from build123d import *

# Parameters (mm, degrees)
SKETCH1_R           = 11
BOSS_EXTRUDE1_DEPTH = 7
SKETCH2_R           = 11
BOSS_EXTRUDE2_DEPTH = 1
SKETCH3_R           = 13.5
SKETCH3_R_2         = 11
BOSS_EXTRUDE3_DEPTH = 1


with BuildPart() as part:
    # Sketch1 → Boss-Extrude1 (new body)
    with BuildSketch(Plane.XY):
        with BuildLine():
            ThreePointArc((0, -13.5), (13.5, 0), (0, 13.5))
            Line((0, 13.5), (-0.244738618, 13.497781411))
            Line((-0.244738618, 13.497781411), (-25, 13.273371546))
            ThreePointArc((-25, 13.273371546), (-38.377486998, -0.287261592), (-24.877625663, -13.726073795))
            Line((-24.877625663, -13.726073795), (-24.632285191, -13.723844279))
            Line((-24.632285191, -13.723844279), (0, -13.5))
        make_face()
        with Locations((-24.877625663, -0.226073795)):
            Circle(SKETCH1_R, mode=Mode.SUBTRACT)
        Circle(SKETCH1_R, mode=Mode.SUBTRACT)
    extrude(amount=BOSS_EXTRUDE1_DEPTH)

    # Sketch2 → Boss-Extrude2 (add)
    with BuildSketch(Plane(origin=(0, 0, 0), x_dir=(-1, 0, 0), z_dir=(0, 0, -1))):
        with Locations((24.877625663, -0.226073795)):
            Circle(SKETCH2_R)
    extrude(amount=-BOSS_EXTRUDE2_DEPTH)

    # Sketch3 → Boss-Extrude3 (add)
    with BuildSketch(Plane.XY.offset(7)):
        with Locations(Location((-24.877625663, -0.226073795, 0), (0, 0, 90.519379929))):
            Circle(SKETCH3_R)
        with Locations(Location((-24.877625663, -0.226073795, 0), (0, 0, 180))):
            Circle(SKETCH3_R_2, mode=Mode.SUBTRACT)
    extrude(amount=BOSS_EXTRUDE3_DEPTH)


solid = part.part
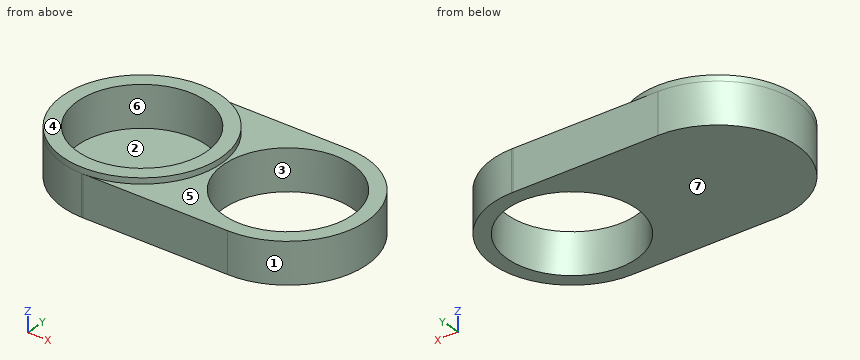
Verification items for the finished model (mm, model axes). Face numbers are marked on the shaded views. A direction names the side the tool comes from. Round coordinates to 2 decimals unless told otherwise and drop trailing zeros. Loops run counter-clockwise (first coordinate to the right, second up) from the corner with the lowest first, then second, coordinate; pieces in that order, holes last. Notation, with made-up numbers: (23.5, 39.25) - (70.5, 39.25) arc R20 cw to (70.5, 46.25) - close; hole circle Ø4 at (31, 71.5). An arc over 180 degrees is marked (long way). Use a Markdown table: item, result. Add a question column.
1. Section check D-D, the plane x = 10. Record the boundary of the cut face in (y, z).
2. Section check A-A, the plane x = -9. Record the boundary of the cut face in (y, z), plus the area to 3 significant figures.
3. Thickness scan on probe 1 along X at (y, z) = (-8.75, 1.25); probe 2 along X at (y, z) = (-1.25, 6.75); probe 3 along X at (y, z) = (0.25, 0.5). Record the ranges inside material, lowest first. Write a range as [from, to].
4. Section check C-C, the plane z = 2. Record the boundary of the cut face in (x, y).
5. Release check for a two-part mould opening along X. For the marked faces 1, 2, 3 and 4 record: released by +X, released by -X, zero draft, split by the parting line, or undercut.
6. Gauge pin test, flat ends, axial feed: pin 1 (1 mm diameter, centred on x = -11.5, z = 2.5, fed in from -Y); pin 2 (1.5 mm diameter, centred on y = -9, z = 4, fed in from +X). Record the tip position at first contact, or that the pin passes through.
7. Access from +Z, -Z, +X, -X, +Y, -Y to the whole of each face (thin tool, end or side, straight path). Record for the marked faces 5, 6 and 7.
8. Section check B-B, the plane y = -10. Record the boundary of the cut face in (x, z), plus the area to 3 significant figures.
Checks:
| question | item | result |
|---|---|---|
| 1 | outline | (-9.07, 0) - (-4.58, 0) - (-4.58, 7) - (-9.07, 7) - close; (4.58, 0) - (9.07, 0) - (9.07, 7) - (4.58, 7) - close |
| 2 | outline | (-13.58, 0) - (-6.32, 0) - (-6.32, 7) - (-13.58, 7) - close; (6.32, 0) - (13.42, 0) - (13.42, 7) - (6.32, 7) - close |
| 2 | area | 100 mm^2 |
| 3 | probe 1 | x = [-35.35, -31.83], [-17.92, -6.67], [6.67, 10.28] |
| 3 | probe 2 | x = [-38.34, -35.83], [-13.93, -10.93], [10.93, 13.44] |
| 3 | probe 3 | x = [-38.37, -11], [11, 13.5] |
| 4 | outline | (-25, 13.27) arc R13.5 ccw to (-24.88, -13.73) - (0, -13.5) arc R13.5 ccw to (0, 13.5) - close; hole circle Ø22 at (-24.88, -0.23); hole circle Ø22 at (0, 0) |
| 5 | face 1 | released by +X |
| 5 | face 2 | undercut |
| 5 | face 3 | undercut |
| 5 | face 4 | zero draft |
| 6 | pin 1 | stops at y = -13.61 |
| 6 | pin 2 | stops at x = 10.69 |
| 7 | face 5 | +Z, +X |
| 7 | face 6 | +Z |
| 7 | face 7 | -Z, +X, -X, +Y, -Y |
| 8 | outline | (-34.19, 0) - (-4.58, 0) - (-4.58, 7) - (-15.57, 7) - (-15.57, 8) - (-19.83, 8) - (-19.83, 1) - (-29.92, 1) - (-29.92, 8) - (-34.19, 8) - close; (4.58, 0) - (9.07, 0) - (9.07, 7) - (4.58, 7) - close |
| 8 | area | 187 mm^2 |
